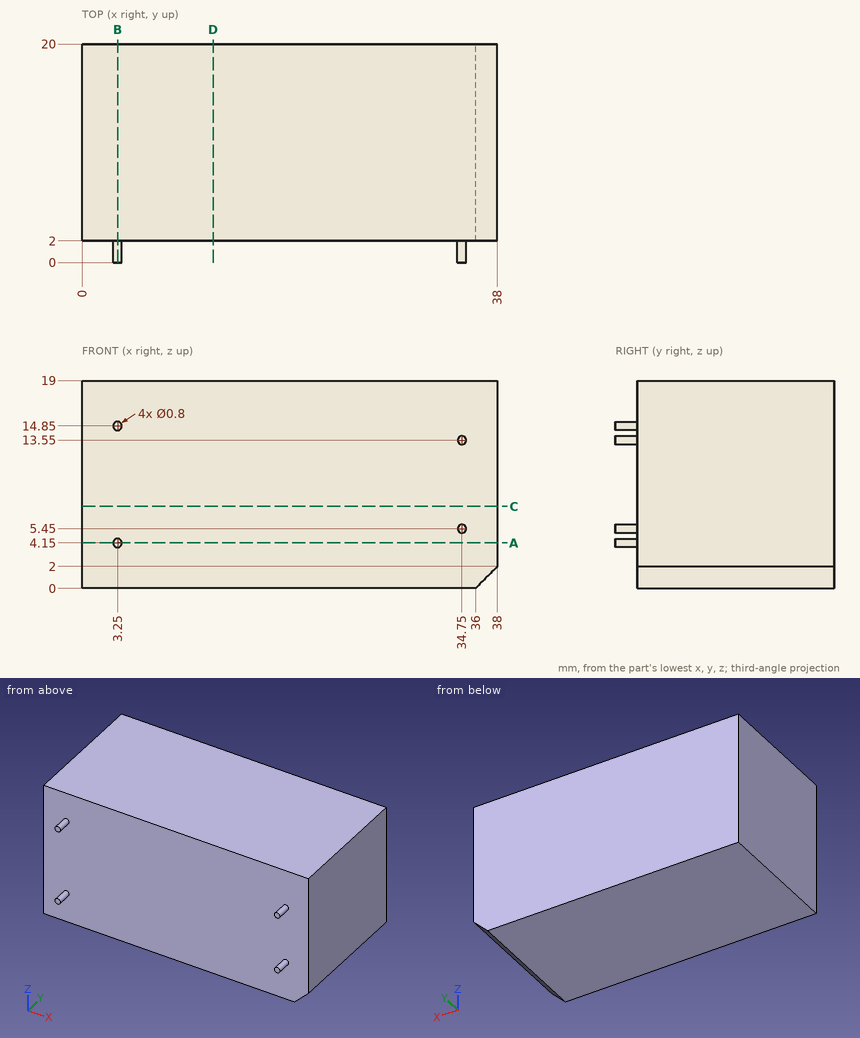
Geometry check sheet. Reference: drawing and pictorial views, mm from the part's lowest x, y, z. Give positions to 0.01 mm unless a question says otherwise; leave off trailing zeros. Loops run counter-clockwise (first coordinate to the right, second up) from the corner with the lowest first, then second, coordinate; pieces in that order, holes last.
1. Section check C-C, the plane z = 7.5. Enter the section's corners in (x, y), then the cut area to 3 significant figures.
2. Section check A-A, the plane z = 4.15. Enter the section's corners in (x, y), then the cut area to 3 significant figures.
3. Section check B-B, the plane x = 3.25. Enter the section's corners in (y, z), then the cut area to 3 significant figures.
4. Go/stop test with flat-tipped pins: pin 1 Ø6 at (x, y) = (17.5, 4.5) entering from -Z; pin 2 Ø9.5 at (x, z) = (10.5, 8) entering from -Y. Record where each tip stops, or that it passes through.
5. Section check D-D, the plane x = 12. Enter the section's corners in (y, z), then the cut area to 3 significant figures.
6. Thickness scan on line 1 (Y direction, x = 32, z = 5); line 2 (X direction, y = 17.75, z = 1.75). Record the ranges inside material, lowest first.
Geometry says:
1. outline: (0, 2) - (38, 2) - (38, 20) - (0, 20) - close
1. area: 684 mm2
2. outline: (0, 2) - (2.85, 2) - (2.85, 0) - (3.65, 0) - (3.65, 2) - (38, 2) - (38, 20) - (0, 20) - close
2. area: 686 mm2
3. outline: (0, 3.75) - (2, 3.75) - (2, 0) - (20, 0) - (20, 19) - (2, 19) - (2, 15.25) - (0, 15.25) - (0, 14.45) - (2, 14.45) - (2, 4.55) - (0, 4.55) - close
3. area: 345 mm2
4. pin 1: stops at z = 0
4. pin 2: stops at y = 2
5. outline: (2, 0) - (20, 0) - (20, 19) - (2, 19) - close
5. area: 342 mm2
6. line 1: y = 2 to 20
6. line 2: x = 0 to 37.75
